Build history of the part. All positions in model axes, mm. A direction names the side the tool comes from. Give positions to 0.01 mm unless a question says otherwise; leave off trailing zeros. Order: outer loops, then holes, each group sorted by start corner. A loop starts at its lowest first (then second) coordinate and runs counter-clockwise, first axis right, second up. Notation, with made-up numbers: M 55,58.5 L 105,58.5 A23 cw 105,81.5 Z; hole C -13.5,78 d3. An arc over 180 degrees is marked long. One line per item, written item: value. Start each with the question number.
from build123d import *

# Parameters (mm, degrees)
SKETCH_1_R          = 2
EXTRUDE_1_DEPTH     = 6
SKETCH_2_R          = 5
SKETCH_2_R_2        = 3.5
CUT_EXTRUDE_1_DEPTH = 0.5
SKETCH_3_R          = 1
CUT_EXTRUDE_2_DEPTH = 5.5


with BuildPart() as part:
    # 草图1 → 凸台-拉伸1 (new body)
    with BuildSketch(Plane.XY):
        Polygon((3.464101615, -6), (6.92820323, 0), (3.464101615, 6), (-3.464101615, 6), (-6.92820323, 0), (-3.464101615, -6), align=None)
        Circle(SKETCH_1_R, mode=Mode.SUBTRACT)
    extrude(amount=EXTRUDE_1_DEPTH)

    # 草图2 → 切除-拉伸1 (cut)
    with BuildSketch(Plane.XY.offset(6)):
        Circle(SKETCH_2_R)
        Circle(SKETCH_2_R_2, mode=Mode.SUBTRACT)
    extrude(amount=-CUT_EXTRUDE_1_DEPTH, mode=Mode.SUBTRACT)

    # 草图3 → 切除-拉伸2 (cut, symmetric)
    with BuildSketch(Plane(origin=(0, 0, 0), x_dir=(-0.8660254037844387, -0.49999999999999983, 0), z_dir=(0.49999999999999983, -0.8660254037844387, 0))):
        Circle(SKETCH_3_R)
    extrude(amount=CUT_EXTRUDE_2_DEPTH, both=True, mode=Mode.SUBTRACT)


solid = part.part
1) Slice it at D-D (z = 0.5). List the corners of the cut face in (x, y).
2) Slice it at C-C (x = 4). List the corners of the cut face in (y, z).
3) Tool access for faces 4 (the flat face through (-5.22, -2.96, 2.96)), 5 (the cylindrical face through (3.233, -1.341, 5.754)), 6 (the flat face through (2.762, -4.756, 0.382)): list every direction of +Z, -Z, +X, -X, +Y, -Y with a clear straight run to the whole face (end or side of a thin tool).
4) Slice it at B-B (z = 2.25). List the corners of the cut face in (x, y).
5) Drop flat-ended pins along their axis: P1, Ø1.5, axis at y = 4.5, z = 4, coming from the +X side; P2, Ø3, axis at y = 0, z = 3.5, coming from the +X side; P3, Ø3, axis at y = -3.5, z = 4, coming from the -X side. Give the stop position or say it passes through.
6) Slice it at A-A (z = 5.75). List the corners of the cut face in (x, y), plus the area to 3 significant figures.
7) Drill centre lines: line 1 (Y direction, x = 0, z = 5.65); line 2 (Y direction, x = 0, z = 2); line 3 (X direction, y = -1.25, z = 5.75). Where is each one in solid material? Low to high.
8) Pull direction Y, two halves, no side cores. Call faces 1 (the flat face through (5.172, -3.042, 2.958)), 2 (the flat face through (-2, -1, 0)), 3 (the flat face through (-2.74, 4.77, 0.38)): pulls with the +Y half, pulls with the -Y half, needs draft (parallel to the pull), parting line crosses it, or undercut.
Results list:
1. outline: M -6.93,0 L -3.46,-6 L 3.46,-6 L 6.93,0 L 3.46,6 L -3.46,6 Z; hole M -3.5,4.33 L -1.65,1.13 A2 ccw 0.15,-1.99 L 2,-5.2 L 3.5,-4.33 L 1.65,-1.13 A2 ccw -0.15,1.99 L -2,5.2 Z
2. outline: M -5.07,0 L 5.07,0 L 5.07,6 L 3,6 L 3,5.5 L -3,5.5 L -3,6 L -5.07,6 Z
3. face 4: +Z, -Z, -X, -Y
3. face 5: +Z
3. face 6: -Z
4. outline: M -6.93,0 L -3.46,-6 L 3.46,-6 L 6.93,0 L 3.46,6 L -3.46,6 Z; hole C 0,0 d4
5. P1: stops at x = 4.76
5. P2: stops at x = 6.93
5. P3: stops at x = -5.77
6. outline: M -6.93,0 L -3.46,-6 L 3.46,-6 L 6.93,0 L 3.46,6 L -3.46,6 Z; C 0,0 d7; hole C 0,0 d10; hole C 0,0 d4
6. area: 72.1 mm²
7. line 1: y = -6 to -5, -3.5 to -2, 2 to 3.5, 5 to 6
7. line 2: y = -6 to -2, 2 to 6
7. line 3: x = -6.21 to -4.84, -3.27 to -1.56, 1.56 to 3.27, 4.84 to 6.21
8. face 1: pulls with the -Y half
8. face 2: needs draft
8. face 3: undercut
